Could you check a few things on this model? Use its own coordinates, in mm. Face numbers are marked on the shaded views. A direction names the side the tool comes from. Coordinates: 2 decimals unless noted, no trailing zeros. Order: outer loops, then holes, each group sorted by start corner. A loop starts at its lowest first (then second) coordinate and runs counter-clockwise, first axis right, second up.
```python
from build123d import *

# Parameters (mm, degrees)
EXTRUDE_1_DEPTH     = 140
SKETCH_2_R          = 12.5
CUT_EXTRUDE_1_DEPTH = 142.955098535
SKETCH_3_R          = 4
CUT_EXTRUDE_2_DEPTH = 138.73356885


with BuildPart() as part:
    # Эскиз1 → Бобышка-Вытянуть1 (new body)
    with BuildSketch(Plane(origin=(0, 0, 0), x_dir=(1, 0, 0), z_dir=(0, 1, 0))):
        with BuildLine():
            Line((-6.992990841, -10.5), (6.992990841, -10.5))
            ThreePointArc((6.992990841, -10.5), (9.472820799, -9.472820799), (10.5, -6.992990841))
            Line((10.5, -6.992990841), (10.5, 6.992990841))
            ThreePointArc((10.5, 6.992990841), (9.472820799, 9.472820799), (6.992990841, 10.5))
            Line((6.992990841, 10.5), (-6.992990841, 10.5))
            ThreePointArc((-6.992990841, 10.5), (-9.472820799, 9.472820799), (-10.5, 6.992990841))
            Line((-10.5, 6.992990841), (-10.5, -6.992990841))
            ThreePointArc((-10.5, -6.992990841), (-9.472820799, -9.472820799), (-6.992990841, -10.5))
        make_face()
        with BuildLine():
            Line((6.5, 8.5), (-6.5, 8.5))
            ThreePointArc((-6.5, 8.5), (-7.914213562, 7.914213562), (-8.5, 6.5))
            Line((-8.5, 6.5), (-8.5, -6.5))
            ThreePointArc((-8.5, -6.5), (-7.914213562, -7.914213562), (-6.5, -8.5))
            Line((-6.5, -8.5), (6.5, -8.5))
            ThreePointArc((6.5, -8.5), (7.914213562, -7.914213562), (8.5, -6.5))
            Line((8.5, -6.5), (8.5, 6.5))
            ThreePointArc((8.5, 6.5), (7.914213562, 7.914213562), (6.5, 8.5))
        make_face(mode=Mode.SUBTRACT)
    extrude(amount=EXTRUDE_1_DEPTH)

    # Эскиз2 → Вырез-Вытянуть1 (cut, through all)
    with BuildSketch(Plane(origin=(0, 0, -10.5), x_dir=(-1, 0, 0), z_dir=(0, 0, -1))):
        with Locations((0, 142.5)):
            Circle(SKETCH_2_R)
    extrude(amount=-CUT_EXTRUDE_1_DEPTH, mode=Mode.SUBTRACT)

    # Эскиз3 → Вырез-Вытянуть2 (cut, through all)
    with BuildSketch(Plane(origin=(10.5, 0, 0), x_dir=(0, 0, -1), z_dir=(1, 0, 0))):
        with Locations((0, 36)):
            Circle(SKETCH_3_R)
        with Locations((0, 61)):
            Circle(SKETCH_3_R)
        with Locations((0, 86)):
            Circle(SKETCH_3_R)
    extrude(amount=-CUT_EXTRUDE_2_DEPTH, mode=Mode.SUBTRACT)


solid = part.part
```
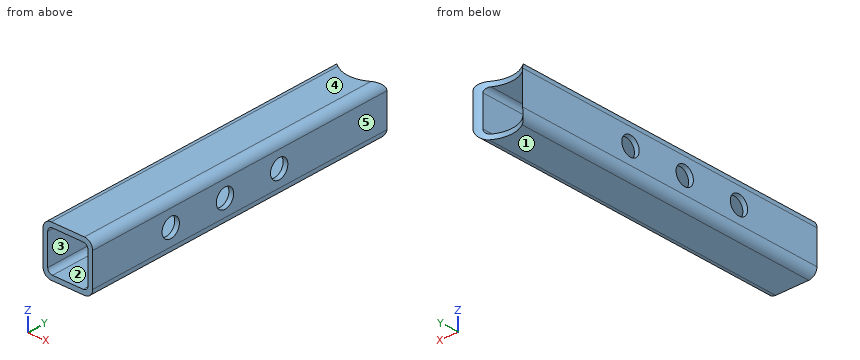
Item 1: I need wall thicknesses on line 1 (Z direction, x = 4.5, y = 65.5); line 2 (Y direction, x = -9.75, z = 0). Which ranges of each line are inside material? Lowest first, please.
Item 2: Suppose I cut it at B-B (x = 0.5). List the corners of the cut face in (y, z) for me, and give its area (3 significant figures).
Item 3: Suppose I cut it at C-C (y = 96). List the corners of the cut face in (x, z) for me.
Item 4: Thinking about a two-plate mould opening in X: for the marked faces 3, 4 and 5, which applies, +X half, -X half, draft (parallel to the pull), parting line (faces both ways), or undercut?
Item 5: Which directions (+Z, -Z, +X, -X, +Y, -Y) give clear straight access to the entire face, cutting with the end or side of a thin tool? Please do the marked faces 1 and 2.
Item 6: Suppose I cut it at D-D (y = 36). List the corners of the cut face in (x, z) for me, and give its area (3 significant figures).
Item 7: Suppose I cut it at A-A (z = 0). Count the separate pieces of the cut face and the enclosed holes in it, and give its area (3 significant figures).
Geometry results:
1. line 1: z = -10.5 to -8.5, 8.5 to 10.5
1. line 2: y = 0 to 32, 40 to 57, 65 to 82, 90 to 134.68
2. outline: (0, -10.5) - (130.01, -10.5) - (130.01, -8.5) - (0, -8.5) - close; (0, 8.5) - (130.01, 8.5) - (130.01, 10.5) - (0, 10.5) - close
2. area: 520 mm2
3. outline: (-10.5, -6.99) arc R3.51 ccw to (-6.99, -10.5) - (6.99, -10.5) arc R3.51 ccw to (10.5, -6.99) - (10.5, 6.99) arc R3.51 ccw to (6.99, 10.5) - (-6.99, 10.5) arc R3.51 ccw to (-10.5, 6.99) - close; hole (-8.5, -6.5) arc R2 ccw to (-6.5, -8.5) - (6.5, -8.5) arc R2 ccw to (8.5, -6.5) - (8.5, 6.5) arc R2 ccw to (6.5, 8.5) - (-6.5, 8.5) arc R2 ccw to (-8.5, 6.5) - close
4. face 3: undercut
4. face 4: draft
4. face 5: +X half
5. face 1: -Z, +X, -X, +Y, -Y
5. face 2: +Y, -Y
6. outline: (-10.5, -6.99) arc R3.51 ccw to (-6.99, -10.5) - (6.99, -10.5) arc R3.51 ccw to (10.5, -6.99) - (10.5, -4) - (8.5, -4) - (8.5, -6.5) arc R2 cw to (6.5, -8.5) - (-6.5, -8.5) arc R2 cw to (-8.5, -6.5) - (-8.5, -4) - (-10.5, -4) - close; (-10.5, 4) - (-8.5, 4) - (-8.5, 6.5) arc R2 cw to (-6.5, 8.5) - (6.5, 8.5) arc R2 cw to (8.5, 6.5) - (8.5, 4) - (10.5, 4) - (10.5, 6.99) arc R3.51 ccw to (6.99, 10.5) - (-6.99, 10.5) arc R3.51 ccw to (-10.5, 6.99) - close
6. area: 113 mm2
7. separate pieces: 8
7. enclosed holes: 0
7. area: 442 mm2
